Design review of the part built by this model. Coordinates are the model's own, in mm. Face numbers are marked on the shaded views. A direction names the side the tool comes from. Give positions to 0.01 mm unless a question says otherwise; leave off trailing zeros. Loops run counter-clockwise (first coordinate to the right, second up) from the corner with the lowest first, then second, coordinate; pieces in that order, holes last. Notation, with made-up numbers: (43, 47) -> (62, 47) arc R36 cw to (62, 82) -> close; hole circle Ø5 at (84, 81). An arc over 180 degrees is marked (long way). Answer in a Markdown table with one row per item. Add a question column.
(1) For the marked faces 1, 2 and 3, list the 3-axis set-ups (+Z, -Z, +X, -X, +Y, -Y) from which the entire face can be reached by the end or side of a thin tool; tool diameter is ignored.
(2) Consider section A-A on y = -12.5. Write out the cut boundary in (x, z).
(3) Consider section D-D on y = -22. Write out the cut boundary in (x, z), then the cut area to 3 significant figures.
(4) For pin 1 (10 mm diameter, centred on x = -0.5, z = 79.5, fed in from -Y); pin 2 (2 mm diameter, centred on y = 11.5, z = 134, fed in from +X); pin 3 (1 mm diameter, centred on y = 13.5, z = 105, fed in from -X), all flat-tipped, find the tip position at first contact; note any pin that passes through.
(5) Consider section C-C on y = 12.5. Write out the cut boundary in (x, z).
(6) Consider section B-B on x = 12.5. Write out the cut boundary in (y, z), then the cut area to 3 significant figures.
(7) For line 1 (Y direction, x = -12.5, z = 9.25); line 2 (Y direction, x = 12, z = 9); line 3 (Z direction, x = -13, y = -25), list the stretches that pass through material, from the lowest coordinate up.
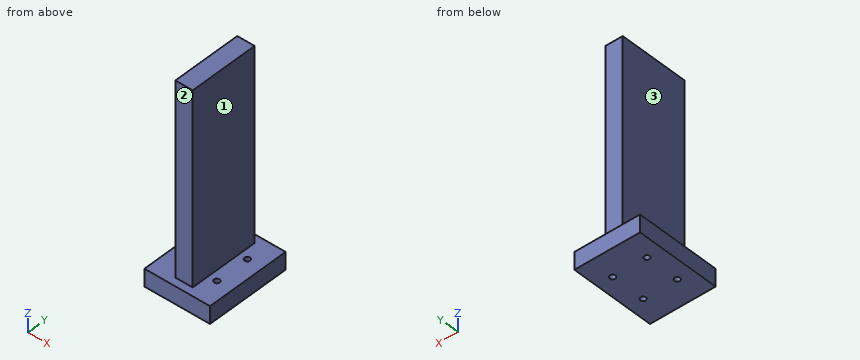
from build123d import *

# Parameters (mm, degrees)
CROQUIS1_W              = 48
CROQUIS1_H              = 62
CROQUIS1_R              = 1.996960485
CROQUIS1_R_2            = 2.003004462
CROQUIS1_R_3            = 2.010116485
CROQUIS1_R_4            = 1.995123233
SALIENTE_EXTRUIR1_DEPTH = 12.7
CROQUIS2_W              = 12.7
CROQUIS2_H              = 50.8
SALIENTE_EXTRUIR2_DEPTH = 140


with BuildPart() as part:
    # Croquis1 → Saliente-Extruir1 (new body)
    with BuildSketch(Plane.XY):
        Rectangle(CROQUIS1_W, CROQUIS1_H)
        with Locations((-12.5, 12.5)):
            Circle(CROQUIS1_R, mode=Mode.SUBTRACT)
        with Locations((12.5, 12.5)):
            Circle(CROQUIS1_R_2, mode=Mode.SUBTRACT)
        with Locations((-12.5, -12.5)):
            Circle(CROQUIS1_R_3, mode=Mode.SUBTRACT)
        with Locations((12.5, -12.5)):
            Circle(CROQUIS1_R_4, mode=Mode.SUBTRACT)
    extrude(amount=SALIENTE_EXTRUIR1_DEPTH)

    # Croquis2 → Saliente-Extruir2 (add)
    with BuildSketch(Plane.XY.offset(12.7)):
        Rectangle(CROQUIS2_W, CROQUIS2_H)
    extrude(amount=SALIENTE_EXTRUIR2_DEPTH)


solid = part.part
Values follow:
| question | item | result |
|---|---|---|
| 1 | face 1 | +Z, +X, +Y, -Y |
| 1 | face 2 | +Z, +X, -X, -Y |
| 1 | face 3 | +Z, -X, +Y, -Y |
| 2 | outline | (-24, 0) -> (-14.51, 0) -> (-14.51, 12.7) -> (-24, 12.7) -> close; (-10.49, 0) -> (10.5, 0) -> (10.5, 12.7) -> (6.35, 12.7) -> (6.35, 152.7) -> (-6.35, 152.7) -> (-6.35, 12.7) -> (-10.49, 12.7) -> close; (14.5, 0) -> (24, 0) -> (24, 12.7) -> (14.5, 12.7) -> close |
| 3 | outline | (-24, 0) -> (24, 0) -> (24, 12.7) -> (6.35, 12.7) -> (6.35, 152.7) -> (-6.35, 152.7) -> (-6.35, 12.7) -> (-24, 12.7) -> close |
| 3 | area | 2,390 mm2 |
| 4 | pin 1 | y = -25.4 |
| 4 | pin 2 | x = 6.35 |
| 4 | pin 3 | x = -6.35 |
| 5 | outline | (-24, 0) -> (-14.5, 0) -> (-14.5, 12.7) -> (-24, 12.7) -> close; (-10.5, 0) -> (10.5, 0) -> (10.5, 12.7) -> (6.35, 12.7) -> (6.35, 152.7) -> (-6.35, 152.7) -> (-6.35, 12.7) -> (-10.5, 12.7) -> close; (14.5, 0) -> (24, 0) -> (24, 12.7) -> (14.5, 12.7) -> close |
| 6 | outline | (-31, 0) -> (-14.5, 0) -> (-14.5, 12.7) -> (-31, 12.7) -> close; (-10.5, 0) -> (10.5, 0) -> (10.5, 12.7) -> (-10.5, 12.7) -> close; (14.5, 0) -> (31, 0) -> (31, 12.7) -> (14.5, 12.7) -> close |
| 6 | area | 686 mm2 |
| 7 | line 1 | -31 to -14.51, -10.49 to 10.5, 14.5 to 31 |
| 7 | line 2 | -31 to -14.43, -10.57 to 10.56, 14.44 to 31 |
| 7 | line 3 | 0 to 12.7 |
